Design review of the part built by this model. Coordinates are the model's own, in mm. Round coordinates to 2 decimals unless told otherwise and drop trailing zeros. Loops run counter-clockwise (first coordinate to the right, second up) from the corner with the lowest first, then second, coordinate; pieces in that order, holes last. Notation, with made-up numbers: (65, -15.75) -> (113, -15.75) arc R22 cw to (113, -8.75) -> close; hole circle Ø8 at (-16.5, -3). An arc over 180 degrees is marked (long way). Answer as CSV lines item,"result". Start each with the question number.
(1) For P1, Ø2, axis at y = -1, z = 14.5, coming from the +X side; P2, Ø2, axis at y = -5.5, z = 21.5, coming from the +X side; P3, Ø5.5, axis at x = -50.45, z = 17.82, coming from the +Y side; P4, Ø1, axis at y = -4.5, z = 11.5, coming from the +X side, all flat-tipped, find the tip position at first contact; note any pin that passes through.
(2) Take a section at A-A, the plane x = 60.5. Write out the cut boundary in (y, z), and give its area (3 significant figures).
(3) Draft analysis for pull direction Z (two halves, no side actions). For faces 1 (the face through (-58.472, -3, 17)), 2 (the face through (-47.929, -3.131, 15.886)), 3 (the face through (-55.9, -3.13, 22.33)), state which applies: +Z half, -Z half, draft (parallel to the pull), parting line (faces both ways), or undercut.
(4) Take a section at B-B, the plane z = 13. Write out the cut boundary in (x, y), and give its area (3 significant figures).
(5) To check wall thickness, follow line 1 (X direction, y = -3, z = 15.5); line 2 (X direction, y = -6, z = 20); line 3 (X direction, y = -4.25, z = 21.25). State the ranges of each line that lie inside material, in increasing order. Write a range as from..to.
(6) Take a section at C-C, the plane y = -2. State how many separate pieces and enclosed holes the cut face has, and give its area (3 significant figures).
from build123d import *

# Parameters (mm, degrees)
F0_W     = 125.926391
F0_H     = 15.030515
F1_DEPTH = 6.35
F2_R     = 5.08
F3_SIZE  = 5.08
F5_D     = 12.7
F7_D     = 6.35


with BuildPart() as f1:
    # F0 (on Front) → F1 (new body)
    with BuildSketch(Plane.XZ):
        with Locations((4.490822, 17.321752)):
            Rectangle(F0_W, F0_H)
    extrude(amount=F1_DEPTH)

    # F2
    f2_edges = [f1.edges().sort_by_distance(p)[0] for p in [
        (67.454018, -3.175, 24.83701),
        (67.454018, -3.175, 9.806495),
    ]]
    fillet(f2_edges, radius=F2_R)

    # F3
    f3_edges = [f1.edges().sort_by_distance(p)[0] for p in [
        (-58.472373, -3.175, 24.83701),
        (-58.472373, -3.175, 9.806495),
    ]]
    chamfer(f3_edges, length=F3_SIZE)

    # F5 (through all)
    with Locations(Plane.XZ.offset(6.35)):
        with Locations((61.007891, 16.751822)):
            Hole(F5_D / 2)

    # F7 (through all)
    with Locations(Plane.XZ.offset(6.35)):
        with Locations((-50.448395, 17.818419)):
            Hole(F7_D / 2)


solid = f1.part
The answers:
1,P1,"x = 67.45"
1,P2,"x = 67.4"
1,P3,"through"
1,P4,"x = 66.55"
2,outline,"(-6.35, 9.81) -> (0, 9.81) -> (0, 10.42) -> (-6.35, 10.42) -> close; (-6.35, 23.08) -> (0, 23.08) -> (0, 24.84) -> (-6.35, 24.84) -> close"
2,area,"15.1 mm²"
3,face 1,"draft"
3,face 2,"undercut"
3,face 3,"+Z half"
4,outline,"(-56.59, -6.35) -> (55.88, -6.35) -> (55.88, 0) -> (-56.59, 0) -> close; (66.13, -6.35) -> (67.09, -6.35) -> (67.09, 0) -> (66.13, 0) -> close"
4,area,"720 mm²"
5,line 1,"-58.47..-52.62, -48.28..54.78, 67.23..67.45"
5,line 2,"-58.23..-52.76, -48.14..55.55, 66.46..67.45"
5,line 3,"-56.98..56.53, 65.49..67.23"
6,separate pieces,"1"
6,enclosed holes,"2"
6,area,"1,700 mm²"
